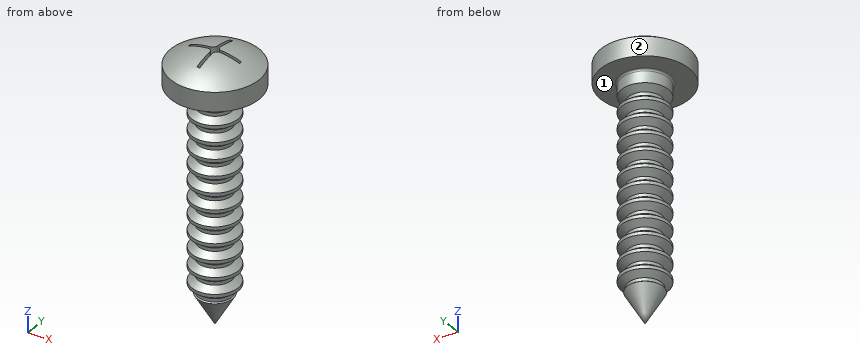
from build123d import *

# Parameters (mm, degrees)
CUT_EXTRUDE_2_DEPTH    = 3.6
PATTERN_LINEAR_1_COUNT = 13
PATTERN_LINEAR_1_PITCH = 2.25
FILLET_1_R             = 0.25


with BuildPart() as part:
    # 草图8 → Revolve 1408 (revolve)
    with BuildSketch(Plane(origin=(0, 0, 0), x_dir=(0, 0, -1), z_dir=(1, 0, 0)), mode=Mode.PRIVATE) as revolve_1408_sk:
        with BuildLine():
            Line((0, 0), (-36.6, 0))
            ThreePointArc((-36.6, 0), (-36.086832981, 3.16227766), (-34.6, 6))
            Line((-34.6, 6), (-32, 6))
            Line((-32, 6), (-32, 3.15))
            Line((-32, 3.15), (-5.455960044, 3.15))
            Line((-5.455960044, 3.15), (0, 0))
        make_face()
    revolve(revolve_1408_sk.sketch.rotate(Axis((0, 0, 11.71), (0, 0, -1)), 90), axis=Axis((0, 0, 11.71), (0, 0, -1)))

    # 草图7 → 切除-拉伸2 (cut)
    with BuildSketch(Plane.XY.offset(36.6)):
        with BuildLine():
            Line((0.2, 3.44419802), (0.2, 0.797500009))
            ThreePointArc((0.2, 0.797500009), (0.375003701, 0.375003701), (0.797500009, 0.2))
            Line((0.797500009, 0.2), (3.44419802, 0.2))
            ThreePointArc((3.44419802, 0.2), (3.45, 0), (3.44419802, -0.2))
            Line((3.44419802, -0.2), (0.797500009, -0.2))
            ThreePointArc((0.797500009, -0.2), (0.375003701, -0.375003701), (0.2, -0.797500009))
            Line((0.2, -0.797500009), (0.2, -3.44419802))
            ThreePointArc((0.2, -3.44419802), (0, -3.45), (-0.2, -3.44419802))
            Line((-0.2, -3.44419802), (-0.2, -0.797500009))
            ThreePointArc((-0.2, -0.797500009), (-0.375003701, -0.375003701), (-0.797500009, -0.2))
            Line((-0.797500009, -0.2), (-3.44419802, -0.2))
            ThreePointArc((-3.44419802, -0.2), (-3.45, 0), (-3.44419802, 0.2))
            Line((-3.44419802, 0.2), (-0.797500009, 0.2))
            ThreePointArc((-0.797500009, 0.2), (-0.375003701, 0.375003701), (-0.2, 0.797500009))
            Line((-0.2, 0.797500009), (-0.2, 3.44419802))
            ThreePointArc((-0.2, 3.44419802), (0, 3.45), (0.2, 3.44419802))
        make_face()
    extrude(amount=-CUT_EXTRUDE_2_DEPTH, mode=Mode.SUBTRACT)

    # 草图9 → 切除-旋转1 (revolve, cut)
    with BuildSketch(Plane(origin=(0, 0, 0), x_dir=(0, 0, -1), z_dir=(1, 0, 0)), mode=Mode.PRIVATE) as cut_revolve_1_sk:
        Polygon((-30.2, 3.15), (-28.4, 3.15), (-29.075, 2.25), (-29.525, 2.25), align=None)
    cut_revolve_1 = revolve(cut_revolve_1_sk.sketch.rotate(Axis((0, 0, 6.911978604), (0, 0, -1)), 90), axis=Axis((0, 0, 6.911978604), (0, 0, -1)), mode=Mode.SUBTRACT)

    # 阵列(线性)1: 切除-旋转1 ×13
    with Locations(*[(0, 0, -i * PATTERN_LINEAR_1_PITCH) for i in range(1, PATTERN_LINEAR_1_COUNT)]):
        add(cut_revolve_1, mode=Mode.SUBTRACT)

    # 圆角1
    fillet_1_edges = [part.edges().sort_by_distance(p)[0] for p in [
        (-3.15, 0, 32),
    ]]
    fillet(fillet_1_edges, radius=FILLET_1_R)


solid = part.part
CAD build for the part. Positions are in the model's coordinates, mm. Face numbers are marked on the shaded views. A direction names the side the tool comes from. Coordinates: 2 decimals unless noted, no trailing zeros. Write each loop counter-clockwise with the first axis right and the second up, starting at its lowest first coordinate (ties: lowest second). Pieces come first, ordered by that corner, then holes. Notation, with made-up numbers: M 37,26 L 73,26 A16 ccw 73,44 Z; hole C 2.5,58.25 d5. An arc over 180 degrees is marked long. Answer as a JSON object with one key per item and string values. Group by question number.
1) Tool access for the marked faces 1 and 2: list every direction of +Z, -Z, +X, -X, +Y, -Y with a clear straight run to the whole face (end or side of a thin tool).
2) Saw through at B-B (y = 4.25). Write the cut outline in (x, z), plus the area to 3 significant figures.
3) Wall check: line 1 (Y direction, x = 1.5, z = 13); line 2 (Y direction, x = -1.25, z = 28); line 3 (Z direction, x = 5.5, y = 1). Give the ranges that are in metal, low to high. Write a range as from..to.
4) Pin check, flat tips, straight feed: pin 1 Ø4 at (y, z) = (2, 18.5) entering from -X; pin 2 Ø2 at (x, z) = (-1.5, 34.5) entering from +Y; pin 3 Ø1 at (x, z) = (-0.5, 4.5) entering from +Y; pin 4 Ø2 at (y, z) = (-4.5, 25.5) entering from -X. Stop position of each tip, or through.
5) Saw through at A-A (y = -4). Write the cut outline in (x, z), plus the area to 3 significant figures.
Values follow:
{
 "1": {"face 1": "-Z", "face 2": "+Z, -Z"},
 "2": {"outline": "M -4.24,32 L 4.24,32 L 4.24,34.6 A9.05 ccw -4.24,34.6 Z", "area": "28.0 mm2"},
 "3": {"line 1": "y = -2.22..2.22", "line 2": "y = -2.89..2.89", "line 3": "z = 32..34.89"},
 "4": {"pin 1": "stops at x = -3.15", "pin 2": "stops at y = 5.98", "pin 3": "stops at y = 2.51", "pin 4": "passes through"},
 "5": {"outline": "M -4.47,32 L 4.47,32 L 4.47,34.6 A9.17 ccw -4.47,34.6 Z", "area": "30.3 mm2"}
}
